Drawing for the job (mm, zero at the part's lowest x, y, z). A direction names the side the tool comes from. Give positions to 0.01 mm unless a question says otherwise; leave off trailing zeros. Order: outer loops, then holes, each group sorted by start corner. A loop starts at its lowest first (then second) coordinate and runs counter-clockwise, first axis right, second up. Notation, with made-up numbers: (-21, 34) -> (-10, 34) arc R33 ccw to (-10, 73) -> close; hole circle Ø7 at (11.25, 38). An arc over 180 degrees is marked (long way). Use one line per item in the form item = value. Start each with the question number.
1) Drop a flat-ended pin along its axis: P1, Ø6, axis at x = 18.5, y = 49, coming from the +Z side. Give the stop position or say it passes through.
2) Cut at B-B, the plane x = 35.5. Give the cut face in (y, z).
3) Cut at C-C, the plane y = 49.5. Give the cut face in (x, z), and give its area (4 significant figures).
4) Probe line 1 (Y direction, x = 49, z = 8.25); line 2 (X direction, y = 10, z = 16.75); line 3 (Z direction, x = 9, y = 40.5). List the from-to ranges inside material, lowest first.
5) Cut at A-A, the plane z = 5.25. Give the cut face in (x, y), and give its area (3 significant figures).
6) Mould opens along X. For the marked faces 1, 2 and 3 say: pulls with the +X half, pulls with the -X half, needs draft (parallel to the pull), parting line crosses it, or undercut.
7) Tool access for the marked faces 4 and 5: list every direction of +Z, -Z, +X, -X, +Y, -Y with a clear straight run to the whole face (end or side of a thin tool).
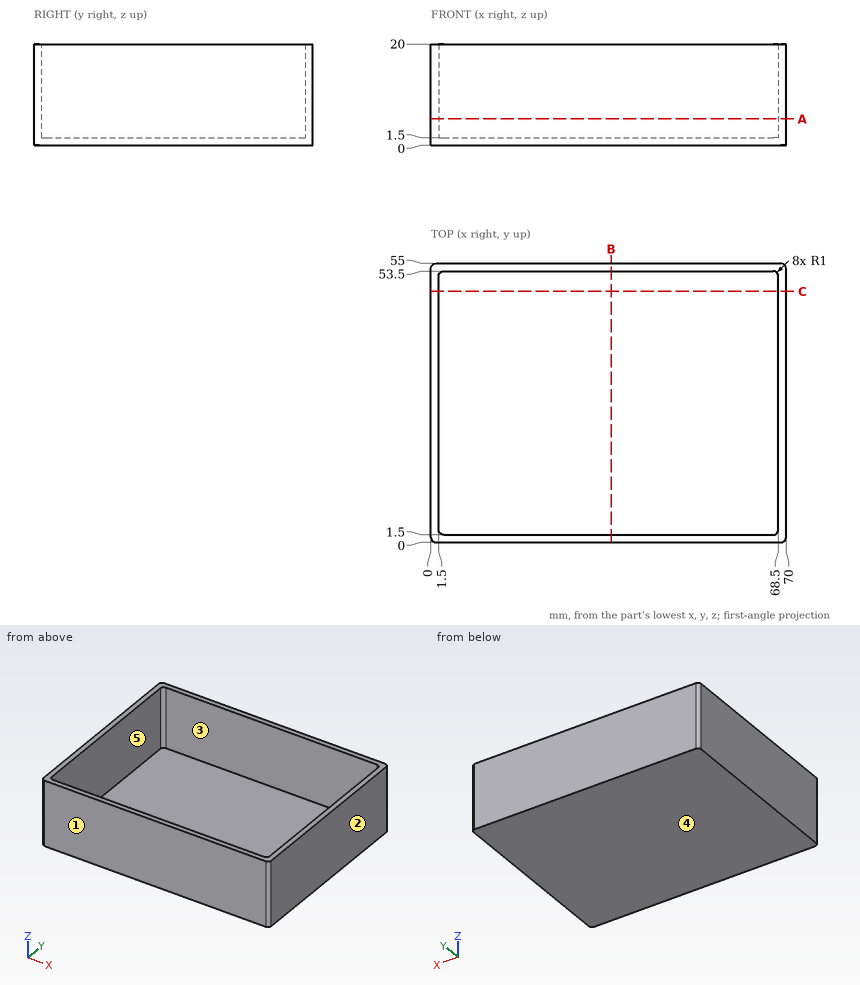
Result:
q1.P1 = 1.5
q2.outline = (0, 0) -> (55, 0) -> (55, 20) -> (53.5, 20) -> (53.5, 1.5) -> (1.5, 1.5) -> (1.5, 20) -> (0, 20) -> close
q3.outline = (0, 0) -> (70, 0) -> (70, 20) -> (68.5, 20) -> (68.5, 1.5) -> (1.5, 1.5) -> (1.5, 20) -> (0, 20) -> close
q3.area = 160.5 mm²
q4.line_1 = 0 to 1.5, 53.5 to 55
q4.line_2 = 0 to 1.5, 68.5 to 70
q4.line_3 = 0 to 1.5
q5.outline = (0, 1) arc R1 ccw to (1, 0) -> (69, 0) arc R1 ccw to (70, 1) -> (70, 54) arc R1 ccw to (69, 55) -> (1, 55) arc R1 ccw to (0, 54) -> close; hole (1.5, 2.5) arc R1 ccw to (2.5, 1.5) -> (67.5, 1.5) arc R1 ccw to (68.5, 2.5) -> (68.5, 52.5) arc R1 ccw to (67.5, 53.5) -> (2.5, 53.5) arc R1 ccw to (1.5, 52.5) -> close
q5.area = 366 mm²
q6.face_1 = needs draft
q6.face_2 = pulls with the +X half
q6.face_3 = undercut
q7.face_4 = -Z, +X, -X, +Y, -Y
q7.face_5 = +Z
